from build123d import *

# Parameters (mm, degrees)
SZKIC1_R                    = 14
SZKIC1_R_2                  = 8.1
DODANIE_WYCI_GNI_CIE1_DEPTH = 3
SZKIC2_R                    = 11
SZKIC2_R_2                  = 8.1
DODANIE_WYCI_GNI_CIE2_DEPTH = 22
SFAZOWANIE1_SIZE            = 0.5


with BuildPart() as part:
    # Szkic1 → Dodanie-wyciągnięcie1 (new body)
    with BuildSketch(Plane(origin=(0, 0, 0), x_dir=(0, 0, -1), z_dir=(1, 0, 0))):
        Circle(SZKIC1_R)
        Circle(SZKIC1_R_2, mode=Mode.SUBTRACT)
    extrude(amount=DODANIE_WYCI_GNI_CIE1_DEPTH)

    # Szkic2 → Dodanie-wyciągnięcie2 (add)
    with BuildSketch(Plane(origin=(3, 0, 0), x_dir=(0, 0, -1), z_dir=(1, 0, 0))):
        Circle(SZKIC2_R)
        Circle(SZKIC2_R_2, mode=Mode.SUBTRACT)
    extrude(amount=DODANIE_WYCI_GNI_CIE2_DEPTH)

    # Sfazowanie1
    sfazowanie1_edges = [part.edges().sort_by_distance(p)[0] for p in [
        (0, 0, 14),
    ]]
    chamfer(sfazowanie1_edges, length=SFAZOWANIE1_SIZE)


solid = part.part
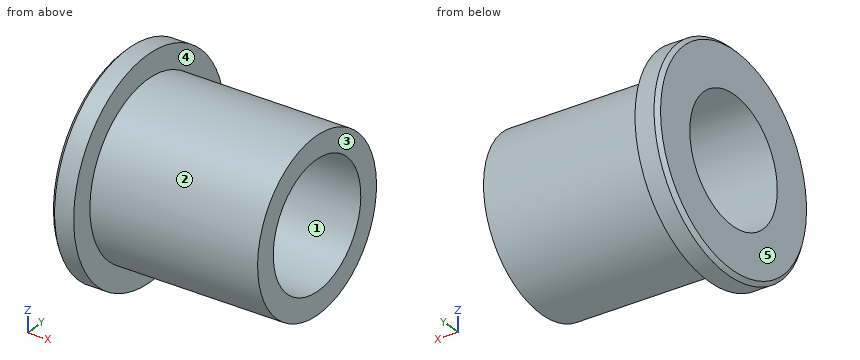
Could you check a few things on this model? Use its own coordinates, in mm. Face numbers are marked on the shaded views. A direction names the side the tool comes from. Coordinates: 2 decimals unless noted, no trailing zeros. Order: outer loops, then holes, each group sorted by start corner. A loop starts at its lowest first (then second) coordinate and runs counter-clockwise, first axis right, second up.
Q1. Will these pins go through, and if not, where does the flat tip stop? pin 1 (1 mm diameter, centred on x = 18.5, z = 4.5, fed in from -Y); pin 2 (14.5 mm diameter, centred on y = 0, z = 0, fed in from -X); pin 3 (12 mm diameter, centred on x = 5.5, z = 11, fed in from -Y); pin 4 (6 mm diameter, centred on x = 18.5, z = 7, fed in from +Y).
Q2. Thinking about a two-plate mould opening in Z: for the marked faces 1, 2 and 3, which applies, released by +Z, released by -Z, zero draft, split by the parting line, or undercut?
Q3. Which directions (+Z, -Z, +X, -X, +Y, -Y) give clear straight access to the entire face, cutting with the end or side of a thin tool? Please do the marked faces 4 and 5.
Q4. Please list where these lines run through material, in increasing order: L1, parallel to Y at x = 7.75, z = 0; L2, parallel to X at y = 10.25, z = -5.75; L3, parallel to Y at x = 11.5, z = -5.5.
Q5. Suppose I cut it at A-A on z = 0. Please give me the cut outline in (x, y).
Q6. Suppose I cut it at C-C on x = 14. Please give me the cut outline in (y, z), and give its area (3 significant figures).
Answer:
1. pin 1: stops at y = -10.25
1. pin 2: passes through
1. pin 3: stops at y = -12.85
1. pin 4: stops at y = 10.25
2. face 1: undercut
2. face 2: split by the parting line
2. face 3: zero draft
3. face 4: +X
3. face 5: +Z, -Z, -X, +Y, -Y
4. L1: y = -11 to -8.1, 8.1 to 11
4. L2: x = 0 to 3
4. L3: y = -9.53 to -5.95, 5.95 to 9.53
5. outline: (0, -13.5) - (0.5, -14) - (3, -14) - (3, -11) - (25, -11) - (25, -8.1) - (0, -8.1) - close; (0, 8.1) - (25, 8.1) - (25, 11) - (3, 11) - (3, 14) - (0.5, 14) - (0, 13.5) - close
6. outline: circle Ø22 at (0, 0); hole circle Ø16.2 at (0, 0)
6. area: 174 mm2
